CAD build for the part. Positions are in the model's coordinates, mm. A direction names the side the tool comes from. Give positions to 0.01 mm unless a question says otherwise; leave off trailing zeros. Write each loop counter-clockwise with the first axis right and the second up, starting at its lowest first coordinate (ties: lowest second). Pieces come first, ordered by that corner, then holes. Notation, with made-up numbers: (57.5, 13) - (105.5, 13) arc R7 ccw to (105.5, 21) - close; hole circle Ø3 at (-33, -17). An arc over 180 degrees is marked (long way). Put each result on its own line as item: value. Start each with the question number.
1. Cut at A-A on z = 0.2. List the corners of the cut face in (x, y), and give its area (3 significant figures).
2. Wall check: line 1 (Y direction, x = 13.75, z = 0.6); line 2 (X direction, y = 11, z = 0.2). Give the ranges that are in metal, low to high.
3. Cut at B-B on x = 3. List the corners of the cut face in (y, z).
4. Drop a flat-ended pin along its axis: pin 1 (3 mm diameter, centred on x = 7.5, y = 11.5, fed in from +Z). Give the stop position or say it passes through.
5. Tool access for faces 1 (the flat face through (0, -3, 0.8)), 2 (the cylindrical face through (-10.6, 15.18, 0.39)): list every direction of +Z, -Z, +X, -X, +Y, -Y with a clear straight run to the whole face (end or side of a thin tool).
6. Mould opens along Y. For faces 3 (the cylindrical face through (10.57, 15.15, 0.39)), 4 (the cylindrical face through (14.21, -14.64, 0.39)), 5 (the flat face through (0, -3, 0)) say: +Y half, -Y half, draft (parallel to the pull), parting line (faces both ways), or undercut.
from build123d import *

# Parameters (mm, degrees)
SKETCH_W     = 31.5
SKETCH_H     = 31.5
SKETCH_R     = 1
PAD_DEPTH    = 0.8
FILLET_R     = 2
SKETCH001_W  = 20
SKETCH001_H  = 7
POCKET_DEPTH = 0.801
FILLET001_R  = 2


with BuildPart() as part:
    # Sketch → Pad (new body)
    with BuildSketch(Plane.XY):
        Rectangle(SKETCH_W, SKETCH_H)
        with Locations((-13.75, 13.75)):
            Circle(SKETCH_R, mode=Mode.SUBTRACT)
        with Locations((13.75, 13.75)):
            Circle(SKETCH_R, mode=Mode.SUBTRACT)
        with Locations((-13.75, -13.75)):
            Circle(SKETCH_R, mode=Mode.SUBTRACT)
        with Locations((13.75, -13.75)):
            Circle(SKETCH_R, mode=Mode.SUBTRACT)
    extrude(amount=PAD_DEPTH)

    # Fillet
    fillet_edges = [part.edges().sort_by_distance(p)[0] for p in [
        (-15.75, 15.75, 0.4),
        (-15.75, -15.75, 0.4),
        (15.75, -15.75, 0.4),
        (15.75, 15.75, 0.4),
    ]]
    fillet(fillet_edges, radius=FILLET_R)

    # Sketch001 (on Face5 of Fillet) → Pocket (cut, through all)
    with BuildSketch(Plane.XY.offset(0.8)):
        with Locations((0, 12.25)):
            Rectangle(SKETCH001_W, SKETCH001_H)
    extrude(amount=-POCKET_DEPTH, mode=Mode.SUBTRACT)

    # Fillet001
    fillet001_edges = [part.edges().sort_by_distance(p)[0] for p in [
        (-10, 15.75, 0.4),
        (-10, 8.75, 0.4),
        (10, 8.75, 0.4),
        (10, 15.75, 0.4),
    ]]
    fillet(fillet001_edges, radius=FILLET001_R)


solid = part.part
Report:
1. outline: (-15.75, -13.75) arc R2 ccw to (-13.75, -15.75) - (13.75, -15.75) arc R2 ccw to (15.75, -13.75) - (15.75, 13.75) arc R2 ccw to (13.75, 15.75) - (12, 15.75) arc R2 ccw to (10, 13.75) - (10, 10.75) arc R2 cw to (8, 8.75) - (-8, 8.75) arc R2 cw to (-10, 10.75) - (-10, 13.75) arc R2 ccw to (-12, 15.75) - (-13.75, 15.75) arc R2 ccw to (-15.75, 13.75) - close; hole circle Ø2 at (-13.75, -13.75); hole circle Ø2 at (-13.75, 13.75); hole circle Ø2 at (13.75, -13.75); hole circle Ø2 at (13.75, 13.75)
1. area: 836 mm²
2. line 1: y = -15.75 to -14.75, -12.75 to 12.75, 14.75 to 15.75
2. line 2: x = -15.75 to -10, 10 to 15.75
3. outline: (-15.75, 0) - (8.75, 0) - (8.75, 0.8) - (-15.75, 0.8) - close
4. pin 1: passes through
5. face 1: +Z, +X, -X, +Y, -Y
5. face 2: +Z, -Z, +Y
6. face 3: +Y half
6. face 4: undercut
6. face 5: draft
